```python
from build123d import *

# Parameters (mm, degrees)
F0_W     = 50.8
F0_H     = 50.8
F1_DEPTH = 25.4
F2_R     = 1.5875
F3_DEPTH = 25.4
F4_R     = 7.9375
F5_T     = -3.81


with BuildPart() as f1:
    # F0 (on Top) → F1 (new body)
    with BuildSketch(Plane.XY):
        Rectangle(F0_W, F0_H)
    extrude(amount=F1_DEPTH)

    # F2 (on face) → F3 (cut, through all)
    with BuildSketch(Plane.XY.offset(25.4)):
        with Locations((17.3482, 17.3482)):
            Circle(F2_R)
        with Locations((17.3482, -17.3482)):
            Circle(F2_R)
        with Locations((-17.3482, 17.3482)):
            Circle(F2_R)
        with Locations((-17.3482, -17.3482)):
            Circle(F2_R)
    extrude(amount=-F3_DEPTH, mode=Mode.SUBTRACT)

    # F4
    f4_edges = [f1.edges().sort_by_distance(p)[0] for p in [
        (25.4, -25.4, 12.7),
        (25.4, 25.4, 12.7),
        (-25.4, -25.4, 12.7),
        (-25.4, 25.4, 12.7),
    ]]
    fillet(f4_edges, radius=F4_R)

    # F5
    f5_openings = [f1.faces().sort_by_distance(p)[0] for p in [
        (0, 0, 25.4),
    ]]
    offset(amount=F5_T, openings=f5_openings, kind=Kind.INTERSECTION)


solid = f1.part
```
Can you work these out from the model? Positions are in its coordinate system, mm. A direction names the side the tool comes from. Round coordinates to 2 decimals unless told otherwise and drop trailing zeros. Loops run counter-clockwise (first coordinate to the right, second up) from the corner with the lowest first, then second, coordinate; pieces in that order, holes last. Notation, with made-up numbers: (-20, 81.25) -> (18, 81.25) arc R25 ccw to (18, 113.25) -> close; hole circle Ø11 at (-34, -17.5). An arc over 180 degrees is marked (long way). One line per item, written item: value. Start each with the question number.
1. If we mould it in two halves opening along Y, with no side actions, what happens to faces 3 (the cylindrical face through (-23.14, -23.01, 12.88)), 4 (the cylindrical face through (-23.14, 23.01, 12.88)), 5 (the cylindrical face through (17.142, -15.774, 12.878))? For each: pulls with the +Y half, pulls with the -Y half, needs draft (parallel to the pull), parting line crosses it, or undercut.
2. For pin 1 (12 mm diameter, centred on x = 14.5, y = 5, fed in from -Z); pin 2 (1.9 mm diameter, centred on x = 17.35, y = -17.35, fed in from +Z); pin 3 (3 mm diameter, centred on x = -3, y = -12, fed in from +Z), each with a flat end and sliding along its axis, tell me the tip position at first contact or that it passes through.
3. If we section it at A-A, the plane x = 6: Write out the boundary of the cut face in (y, z), then the cut area to 3 significant figures.
4. If we section it at D-D, the plane z = 2.5: Write out the boundary of the cut face in (x, y) (1 decimal), then the cut area to 3 significant figures.
5. For faces 1 (the flat face through (0, 0, 3.81)), 2 (the flat face through (22, 0, 25.4)), which set-ups out of +Z, -Z, +X, -X, +Y, -Y let a thin tool reach every point of the face, with its end or its side?
6. If we section it at C-C, the plane z = 9.5: Write out the boundary of the cut face in (x, y) (1 decimal), then the cut area to 3 significant figures.
7. If I drill on probe 1 along Y at (x, z) = (1, 23.5); probe 2 along Y at (x, z) = (13, 6.5), over which ranges is the centre line in solid material (lowest first)?
Calculated:
1. face 3: pulls with the -Y half
1. face 4: pulls with the +Y half
1. face 5: undercut
2. pin 1: stops at z = 0
2. pin 2: passes through
2. pin 3: stops at z = 3.81
3. outline: (-25.4, 0) -> (25.4, 0) -> (25.4, 25.4) -> (21.59, 25.4) -> (21.59, 3.81) -> (-21.59, 3.81) -> (-21.59, 25.4) -> (-25.4, 25.4) -> close
3. area: 358 mm²
4. outline: (-25.4, -17.5) arc R7.9 ccw to (-17.5, -25.4) -> (17.5, -25.4) arc R7.9 ccw to (25.4, -17.5) -> (25.4, 17.5) arc R7.9 ccw to (17.5, 25.4) -> (-17.5, 25.4) arc R7.9 ccw to (-25.4, 17.5) -> close; hole circle Ø3.2 at (-17.3, -17.3); hole circle Ø3.2 at (-17.3, 17.3); hole circle Ø3.2 at (17.3, -17.3); hole circle Ø3.2 at (17.3, 17.3)
4. area: 2,490 mm²
5. face 1: +Z
5. face 2: +Z, +X, -X, +Y, -Y
6. outline: (-25.4, -17.5) arc R7.9 ccw to (-17.5, -25.4) -> (17.5, -25.4) arc R7.9 ccw to (25.4, -17.5) -> (25.4, 17.5) arc R7.9 ccw to (17.5, 25.4) -> (-17.5, 25.4) arc R7.9 ccw to (-25.4, 17.5) -> close; hole (-21.6, -14) arc R5.4 cw (long way) to (-14, -21.6) -> (14, -21.6) arc R5.4 cw (long way) to (21.6, -14) -> (21.6, 14) arc R5.4 cw (long way) to (14, 21.6) -> (-14, 21.6) arc R5.4 cw (long way) to (-21.6, 14) -> close; hole circle Ø3.2 at (-17.3, -17.3); hole circle Ø3.2 at (-17.3, 17.3); hole circle Ø3.2 at (17.3, -17.3); hole circle Ø3.2 at (17.3, 17.3)
6. area: 956 mm²
7. probe 1: y = -25.4 to -21.59, 21.59 to 25.4
7. probe 2: y = -25.4 to -21.59, -20.55 to -14.15, 14.15 to 20.55, 21.59 to 25.4
